```python
from build123d import *

# Parameters (mm, degrees)
SKETCH1_W           = 53
SKETCH1_H           = 95
BOSS_EXTRUDE1_DEPTH = 5
SKETCH2_R           = 5.5
SKETCH2_R_2         = 1.85
BOSS_EXTRUDE2_DEPTH = 51.5
SKETCH4_R           = 7.5
SKETCH4_R_2         = 2.125
CUT_EXTRUDE1_DEPTH  = 6


with BuildPart() as part:
    # Sketch1 → Boss-Extrude1 (new body)
    with BuildSketch(Plane(origin=(0, 0, 0), x_dir=(1, 0, 0), z_dir=(0, 1, 0))):
        with Locations((26.5, 47.5)):
            Rectangle(SKETCH1_W, SKETCH1_H)
    extrude(amount=BOSS_EXTRUDE1_DEPTH)

    # Sketch2 → Boss-Extrude2 (add)
    with BuildSketch(Plane(origin=(0, 5, 0), x_dir=(1, 0, 0), z_dir=(0, 1, 0))):
        with Locations((46.5, 89.5)):
            Circle(SKETCH2_R)
        with Locations((46.5, 89.5)):
            Circle(SKETCH2_R_2, mode=Mode.SUBTRACT)
        with Locations((6.5, 89.5)):
            Circle(SKETCH2_R)
        with Locations((6.5, 89.5)):
            Circle(SKETCH2_R_2, mode=Mode.SUBTRACT)
        with Locations((6.5, 5.5)):
            Circle(SKETCH2_R)
        with Locations((6.5, 5.5)):
            Circle(SKETCH2_R_2, mode=Mode.SUBTRACT)
        with Locations((46.5, 5.5)):
            Circle(SKETCH2_R)
        with Locations((46.5, 5.5)):
            Circle(SKETCH2_R_2, mode=Mode.SUBTRACT)
    extrude(amount=BOSS_EXTRUDE2_DEPTH)

    # Sketch4 → Cut-Extrude1 (cut, through all)
    with BuildSketch(Plane(origin=(0, 5, 0), x_dir=(1, 0, 0), z_dir=(0, 1, 0))):
        with Locations((26.5, 47.5)):
            Circle(SKETCH4_R)
        with Locations((11.5, 72.5)):
            Circle(SKETCH4_R_2)
        with Locations((41.5, 72.5)):
            Circle(SKETCH4_R_2)
        with Locations((11.5, 22.5)):
            Circle(SKETCH4_R_2)
        with Locations((41.5, 22.5)):
            Circle(SKETCH4_R_2)
    extrude(amount=-CUT_EXTRUDE1_DEPTH, mode=Mode.SUBTRACT)


solid = part.part
```
The model under review builds one solid part; all positions refer to its coordinate system, in mm. A direction names the side the tool comes from. Give positions to 0.01 mm unless a question says otherwise; leave off trailing zeros. Loops run counter-clockwise (first coordinate to the right, second up) from the corner with the lowest first, then second, coordinate; pieces in that order, holes last. Notation, with made-up numbers: (59, 48.5) - (87, 48.5) arc R25 ccw to (87, 67.5) - close; hole circle Ø1 at (25.25, 73). An arc over 180 degrees is marked (long way). Answer as a JSON object with one key per item and string values.
Q1. Add section B-B on y = 20.5. State the section outline as (x, z) points.
Worked out:
{"outline": "circle Ø11 at (6.5, -89.5); circle Ø11 at (6.5, -5.5); circle Ø11 at (46.5, -89.5); circle Ø11 at (46.5, -5.5); hole circle Ø3.7 at (6.5, -89.5); hole circle Ø3.7 at (6.5, -5.5); hole circle Ø3.7 at (46.5, -89.5); hole circle Ø3.7 at (46.5, -5.5)"}
Q2. For faces 4 (the flat face through (46, 5, -6)), 5 (the flat face through (53, 2, -47)), list the 3-axis set-ups (+Z, -Z, +X, -X, +Y, -Y) from which the entire face can be reached by the end or side of a thin tool; tool diameter is ignored.
Worked out:
{"face 4": "+Y", "face 5": "+Z, -Z, +X, +Y, -Y"}
Q3. Insertion check: pin 1 (3 mm diameter, centred on x = 42, y = 35, fed in from -Z); pin 2 (8 mm diameter, centred on x = 47.5, z = -64, fed in from +Y); pin 3 (3 mm diameter, centred on x = 12, y = 39.5, fed in from -Z). Each pin has a flat end and moves straight along its axis. Give the tip position at first contact, or say it passes through.
Worked out:
{"pin 1": "stops at z = -94.11", "pin 2": "stops at y = 5", "pin 3": "stops at z = -93.27"}
Q4. Add section A-A on z = -47.5. State the section outline as (x, y) points.
Worked out:
{"outline": "(0, 0) - (19, 0) - (19, 5) - (0, 5) - close; (34, 0) - (53, 0) - (53, 5) - (34, 5) - close"}
Q5. Add section D-D on z = -22.5. State the section outline as (x, y) points (3 decimals).
Worked out:
{"outline": "(0, 0) - (9.375, 0) - (9.375, 5) - (0, 5) - close; (13.625, 0) - (39.375, 0) - (39.375, 5) - (13.625, 5) - close; (43.625, 0) - (53, 0) - (53, 5) - (43.625, 5) - close"}
Q6. To check wall thickness, follow line 1 along Z through (x, y) = (11.5, 3.6) (3 decimals); line 2 along Z through (x, y) = (46.5, 32.5); line 3 along X through (y, z) = (16.5, -5.5). State the ranges of each line that lie inside material, in increasing order.
Worked out:
{"line 1": "z = -95 to -74.625, -70.375 to -24.625, -20.375 to 0", "line 2": "z = -95 to -91.35, -87.65 to -84, -11 to -7.35, -3.65 to 0", "line 3": "x = 1 to 4.65, 8.35 to 12, 41 to 44.65, 48.35 to 52"}
Q7. Mouldability with a two-part tool opening along Z and no side actions: class faces 1 (the flat face through (26, 2, 0)), 2 (the flat face through (46, 56.5, -3)), 3 (the flat face through (6, 5, -6)) as +Z half, -Z half, draft (parallel to the pull), parting line (faces both ways), or undercut.
Worked out:
{"face 1": "+Z half", "face 2": "draft", "face 3": "undercut"}
Q8. Add section C-C on x = 20. State the section outline as (y, z) points.
Worked out:
{"outline": "(0, -95) - (5, -95) - (5, -51.24) - (0, -51.24) - close; (0, -43.76) - (5, -43.76) - (5, 0) - (0, 0) - close"}
